Geometry: final body of the model. Coordinates: model frame, mm. Face numbers are marked on the shaded views. Give positions to 0.01 mm unless a question says otherwise; leave off trailing zeros. Write each loop counter-clockwise with the first axis right and the second up, starting at its lowest first coordinate (ties: lowest second). Pieces come first, ordered by that corner, then holes. Notation, with made-up numbers: M -8.5,82.25 L 43.5,82.25 A18 cw 43.5,100.25 Z; hole C -5,58 d4. An arc over 180 degrees is marked long. Use one line per item in the form item = value. Start each with the question number.
Item 1: Section query D-D on x = 8.75. Return loops of the section in (y, z).
Item 2: Material intervals for line 1 along X through (y, z) = (-10.5, 7.25); line 2 along Y through (x, z) = (-4.75, 6.5); line 3 along X through (y, z) = (-15.5, 5), sorted ascending. Write a range as from..to.
Item 3: Section query A-A on x = 0. Return loops of the section in (y, z).
Item 4: Contact query for flat-ended pins moving along their axis: P1, Ø6, axis at x = 0.5, y = -4, coming from the +Z side; P2, Ø6, axis at x = -5.5, z = 9, coming from the -Y side. Output: stop coordinate, or through.
Item 5: Section query B-B on y = -15. Return loops of the section in (x, z).
Item 6: Pull-direction query (Y, two-part tool) for the marked faces 1, 2 and 3; classes: released by +Y, released by -Y, zero draft, split by the parting line, or undercut.
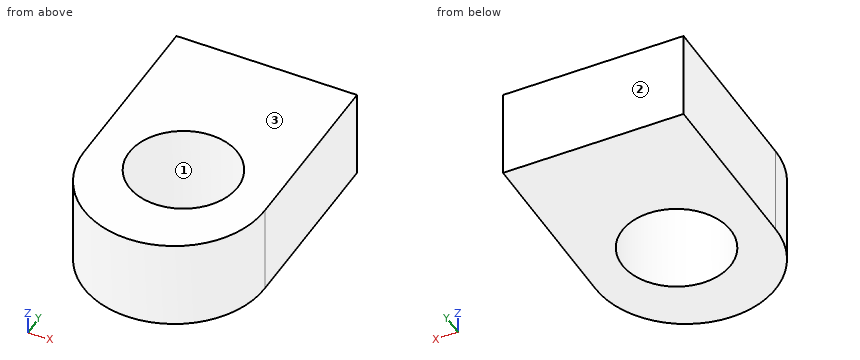
from build123d import *

# Parameters (mm, degrees)
F0_W     = 25.4
F0_H     = 25.4
F1_DEPTH = 12.7
F2_R     = 12.7
F3_DEPTH = 12.7
F4_R     = 7.62
F5_DEPTH = 12.701


with BuildPart() as f1:
    # F0 (on Top) → F1 (new body)
    with BuildSketch(Plane.XY):
        Rectangle(F0_W, F0_H)
    extrude(amount=F1_DEPTH)

    # F2 (on Top) → F3 (join)
    with BuildSketch(Plane.XY):
        with Locations((0, -12.758351)):
            Circle(F2_R)
    extrude(amount=F3_DEPTH)

    # F4 (on face) → F5 (cut, through all)
    with BuildSketch(Plane.XY.offset(12.7)):
        with Locations((0, -10.247545)):
            Circle(F4_R)
    extrude(amount=-F5_DEPTH, mode=Mode.SUBTRACT)


solid = f1.part
Answer sheet:
q1.outline = M -21.96,0 L 12.7,0 L 12.7,12.7 L -21.96,12.7 Z
q2.line_1 = -12.7..-7.62, 7.62..12.7
q2.line_2 = -24.54..-16.21, -4.29..12.7
q2.line_3 = -12.4..-5.52, 5.52..12.4
q3.outline = M -25.46,0 L -17.87,0 L -17.87,12.7 L -25.46,12.7 Z; M -2.63,0 L 12.7,0 L 12.7,12.7 L -2.63,12.7 Z
q4.P1 = 12.7
q4.P2 = -25.21
q5.outline = M -12.5,0 L -5.96,0 L -5.96,12.7 L -12.5,12.7 Z; M 5.96,0 L 12.5,0 L 12.5,12.7 L 5.96,12.7 Z
q6.face_1 = undercut
q6.face_2 = released by +Y
q6.face_3 = zero draft
